Source: CAD feature listing. Evaluate the final solid. Frame: model axes, mm. Give positions to 0.01 mm unless a question says otherwise; leave off trailing zeros. Loops run counter-clockwise (first coordinate to the right, second up) from the corner with the lowest first, then second, coordinate; pieces in that order, holes last. Notation, with made-up numbers: (16, -6) -> (39, -6) arc R26 cw to (39, 27) -> close; hole circle Ø1 at (21.5, 11.25). An arc over 180 degrees is marked (long way). Answer as a JSON object with one key per item and string values. Group by question number.
from build123d import *

# Parameters (mm, degrees)
F0_W     = 100
F0_H     = 100
F1_DEPTH = 5
F2_R     = 5
F3_DEPTH = 5.001


with BuildPart() as f1:
    # F0 (on Front) → F1 (new body)
    with BuildSketch(Plane.XZ):
        with Locations((50, 50)):
            Rectangle(F0_W, F0_H)
    extrude(amount=F1_DEPTH)

    # F2 (on face) → F3 (cut, through all)
    with BuildSketch(Plane.XZ.offset(5)):
        with Locations((15, 85)):
            Circle(F2_R)
        with Locations((85, 85)):
            Circle(F2_R)
        with Locations((15, 15)):
            Circle(F2_R)
        with Locations((85, 15)):
            Circle(F2_R)
    extrude(amount=-F3_DEPTH, mode=Mode.SUBTRACT)


solid = f1.part
(1) First-contact query: pin 1 (8 mm diameter, centred on x = 15, z = 85, fed in from +Y). Flat tip, straight axial feed; report the tip coordinate or a pass-through.
(2) Section query B-B on x = 15. Return the cut outline in (y, z), plus the area to 3 significant figures.
(3) Section query A-A on y = -2.55. Return the cut outline in (x, z).
(4) Material intervals for line 1 (X direction, y = -2.55, z = 85.5); line 2 (Z direction, x = 85, y = -1.2), sorted ascending. Write a range as from..to.
(5) Mould query, pull axis Z, two halves, no side actions, for faces 1 (the face through (100, -2, 49)), 2 (the face through (49, -2, 0)), 3 (the face through (17.307, -2.535, 10.564)), 4 (the face through (49, -2, 100)). Classes: pulls with the +Z half, pulls with the -Z half, needs draft (parallel to the pull), parting line crosses it, or undercut.
(6) Section query C-C on z = 85. Return the cut outline in (x, y).
Result:
{
 "1": {"pin 1": "through"},
 "2": {"outline": "(-5, 0) -> (0, 0) -> (0, 10) -> (-5, 10) -> close; (-5, 20) -> (0, 20) -> (0, 80) -> (-5, 80) -> close; (-5, 90) -> (0, 90) -> (0, 100) -> (-5, 100) -> close", "area": "400 mm²"},
 "3": {"outline": "(0, 0) -> (100, 0) -> (100, 100) -> (0, 100) -> close; hole circle Ø10 at (15, 15); hole circle Ø10 at (15, 85); hole circle Ø10 at (85, 15); hole circle Ø10 at (85, 85)"},
 "4": {"line 1": "0..10.03, 19.97..80.03, 89.97..100", "line 2": "0..10, 20..80, 90..100"},
 "5": {"face 1": "needs draft", "face 2": "pulls with the -Z half", "face 3": "undercut", "face 4": "pulls with the +Z half"},
 "6": {"outline": "(0, -5) -> (10, -5) -> (10, 0) -> (0, 0) -> close; (20, -5) -> (80, -5) -> (80, 0) -> (20, 0) -> close; (90, -5) -> (100, -5) -> (100, 0) -> (90, 0) -> close"}
}
